from build123d import *

# Parameters (mm, degrees)
SKETCH2_W           = 113.13708499
SKETCH2_H           = 113.13708499
BOSS_EXTRUDE1_DEPTH = 3.5
CHAMFER1_SIZE       = 2.5
BOSS_EXTRUDE3_DEPTH = 15
BOSS_EXTRUDE5_DEPTH = 15
CIRPATTERN11_COUNT  = 4
CUT_EXTRUDE3_START  = -18.5
SKETCH8_R           = 1.5
CUT_EXTRUDE3_DEPTH  = 18.5
SKETCH9_R           = 3.603183746
CUT_EXTRUDE4_DEPTH  = 10


with BuildPart() as part:
    # Sketch2 → Boss-Extrude1 (new body)
    with BuildSketch(Plane(origin=(0, 0, 0), x_dir=(1, 0, 0), z_dir=(0, 1, 0))):
        Rectangle(SKETCH2_W, SKETCH2_H)
    extrude(amount=BOSS_EXTRUDE1_DEPTH)

    # Chamfer1
    chamfer1_edges = [part.edges().sort_by_distance(p)[0] for p in [
        (56.568542495, 1.75, 56.568542495),
        (-56.568542495, 1.75, 56.568542495),
        (-56.568542495, 1.75, -56.568542495),
        (56.568542495, 1.75, -56.568542495),
    ]]
    chamfer(chamfer1_edges, length=CHAMFER1_SIZE)

    # Sketch3 → Boss-Extrude3 (add)
    with BuildSketch(Plane.XZ):
        Polygon((0, 10.253048327), (-3.535533906, 6.717514421), (0, 3.181980515), (3.535533906, 6.717514421), align=None)
        Polygon((-21.213203436, 24.395183951), (-3.535533906, 6.717514421), (0, 10.253048327), (-17.67766953, 27.930717857), align=None)
        Polygon((17.67766953, 27.930717857), (0, 10.253048327), (3.535533906, 6.717514421), (21.213203436, 24.395183951), align=None)
        Polygon((6.717514421, 3.535533906), (3.181980515, 0), (6.717514421, -3.535533906), (10.253048327, 0), align=None)
        Polygon((24.395183951, 21.213203436), (6.717514421, 3.535533906), (10.253048327, 0), (27.930717857, 17.67766953), align=None)
        Polygon((10.253048327, 0), (6.717514421, -3.535533906), (24.395183951, -21.213203436), (27.930717857, -17.67766953), align=None)
        Polygon((3.535533906, -6.717514421), (0, -3.181980515), (-3.535533906, -6.717514421), (0, -10.253048327), align=None)
        Polygon((21.213203436, -24.395183951), (3.535533906, -6.717514421), (0, -10.253048327), (17.67766953, -27.930717857), align=None)
        Polygon((0, -10.253048327), (-3.535533906, -6.717514421), (-21.213203436, -24.395183951), (-17.67766953, -27.930717857), align=None)
        Polygon((-6.717514421, -3.535533906), (-3.181980515, 0), (-6.717514421, 3.535533906), (-10.253048327, 0), align=None)
        Polygon((-24.395183951, -21.213203436), (-6.717514421, -3.535533906), (-10.253048327, 0), (-27.930717857, -17.67766953), align=None)
        Polygon((-10.253048327, 0), (-6.717514421, 3.535533906), (-24.395183951, 21.213203436), (-27.930717857, 17.67766953), align=None)
    extrude(amount=BOSS_EXTRUDE3_DEPTH)

    # Sketch6 → Boss-Extrude5 (add)
    with BuildSketch(Plane(origin=(0, 3.5, 0), x_dir=(1, 0, 0), z_dir=(0, 1, 0))):
        Polygon((-66.949331771, 70.131312286), (-42.20059443, 45.382574945), (-38.665060524, 48.918108851), (-63.413797865, 73.666846192), align=None)
        Polygon((-45.382574945, 42.20059443), (-48.918108851, 38.665060524), (-73.666846192, 63.413797865), (-70.131312286, 66.949331771), align=None)
    boss_extrude5 = extrude(amount=BOSS_EXTRUDE5_DEPTH)

    # CirPattern11: Boss-Extrude5 ×4 about axis
    cirpattern11_axis = Axis((0.511078202, 0, 0.511078202), (0, 1, 0))
    for i in range(1, CIRPATTERN11_COUNT):
        add(boss_extrude5.rotate(cirpattern11_axis, i * 360 / CIRPATTERN11_COUNT))

    # Sketch8 → Cut-Extrude3 (cut)
    with BuildSketch(Plane(origin=(0, 3.5, 0), x_dir=(1, 0, 0), z_dir=(0, 1, 0)).offset(CUT_EXTRUDE3_START)):
        with Locations(Location((0, 10.5, 0), (0, 0, 270))):
            Circle(SKETCH8_R)
        with Locations(Location((0, -10.5, 0), (0, 0, 270))):
            Circle(SKETCH8_R)
        with Locations(Location((0, 17.5, 0), (0, 0, 270))):
            Circle(SKETCH8_R)
        with Locations(Location((0, -17.5, 0), (0, 0, 270))):
            Circle(SKETCH8_R)
    extrude(amount=CUT_EXTRUDE3_DEPTH, mode=Mode.SUBTRACT)

    # Sketch9 → Cut-Extrude4 (cut)
    with BuildSketch(Plane.XZ):
        with Locations((0, 10.5)):
            Circle(SKETCH9_R)
        with Locations((0, -10.5)):
            Circle(SKETCH9_R)
    extrude(amount=CUT_EXTRUDE4_DEPTH, mode=Mode.SUBTRACT)


solid = part.part
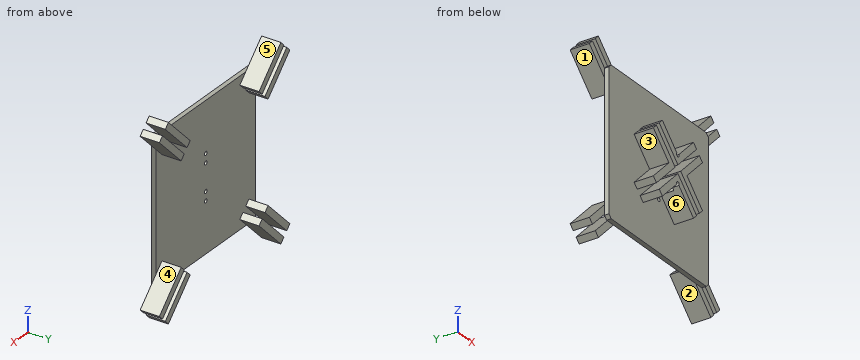
Read the model definition and answer for the solid it produces. Units are mm, in the model's axes. Face numbers are marked on the shaded views. A direction names the side the tool comes from. Round coordinates to 2 decimals unless told otherwise and drop trailing zeros. Write each loop counter-clockwise with the first axis right and the second up, starting at its lowest first coordinate (ties: lowest second). Pieces come first, ordered by that corner, then holes.
Q1. Find section C-C on x = -13.5. Determine the outline of the cut face in (y, z), and give its area (3 significant figures).
Values:
outline: (-15, -23.75) - (0, -23.75) - (0, -56.57) - (3.5, -56.57) - (3.5, 56.57) - (0, 56.57) - (0, 23.75) - (-15, 23.75) - (-15, 16.68) - (0, 16.68) - (0, 10.32) - (-15, 10.32) - (-15, 3.25) - (0, 3.25) - (0, -3.25) - (-15, -3.25) - (-15, -10.32) - (0, -10.32) - (0, -16.68) - (-15, -16.68) - close
area: 820 mm2
Q2. Straight lines are drawn through the part: line 1 (Z direction, x = 0, y = 1); line 2 (Z direction, x = -20.5, y = -3.5); line 3 (X direction, y = -4, z = 10). For each, find the intervals that lie inside material, in ascending order.
Values:
line 1: z = -56.57 to -19, -16 to -12, -9 to 9, 12 to 16, 19 to 56.57
line 2: z = -25.11 to -23.68, -17.32 to -10.25, 10.25 to 17.32, 23.68 to 25.11
line 3: x = -20.25 to -13.18, -6.82 to -3.57, 3.57 to 6.82, 13.18 to 20.25
Q3. Find section D-D on x = -34. Determine the outline of the cut face in (y, z).
Values:
outline: (0, -56.57) - (3.5, -56.57) - (3.5, 56.57) - (0, 56.57) - close
Q4. A tool of negligible diameter and unlimited length cuts with its end or side. For the marked faces 1, 2 and 3, from which of +Z, -Z, +X, -X, +Y, -Y can it reach the whole face along a straight path? Write none if from no direction.
Values:
face 1: -X, +Y
face 2: -Z, +Y
face 3: -X, -Y
Q5. Flat-ended cylindrical pins translate along their axes: P1, Ø1.5, axis at x = -22, z = -32, coming from the +Y side; P2, Ø10, axis at x = -36.5, y = 6, coming from the -Z side; P3, Ø4, axis at y = 3, z = 1, coming from the -X side. Find the tip coordinate at first contact, or state that the pin passes through.
Values:
P1: stops at y = 3.5
P2: stops at z = -56.57
P3: stops at x = -56.57
Q6. The mould has two halves that part along Z. Classify the marked faces 4, 5 and 6: released by +Z, released by -Z, zero draft, split by the parting line, or undercut.
Values:
face 4: undercut
face 5: released by +Z
face 6: released by -Z
Q7. Find section B-B on y = -7.5. Determine the outline of the cut face in (x, z).
Values:
outline: (-27.93, -17.68) - (-24.4, -21.21) - (-3.18, 0) - (-24.4, 21.21) - (-27.93, 17.68) - (-10.25, 0) - close; (-21.21, -24.4) - (-17.68, -27.93) - (-2.67, -12.92) arc R3.6 cw (long way) to (2.67, -12.92) - (17.68, -27.93) - (21.21, -24.4) - (0, -3.18) - close; (-21.21, 24.4) - (0, 3.18) - (21.21, 24.4) - (17.68, 27.93) - (2.67, 12.92) arc R3.6 cw (long way) to (-2.67, 12.92) - (-17.68, 27.93) - close; (3.18, 0) - (24.4, -21.21) - (27.93, -17.68) - (10.25, 0) - (27.93, 17.68) - (24.4, 21.21) - close
Q8. Find section A-A on y = 15.5. State how many separate pieces and enclosed holes the cut face has, and give its area (3 significant figures).
Values:
separate pieces: 8
enclosed holes: 0
area: 1,400 mm2
